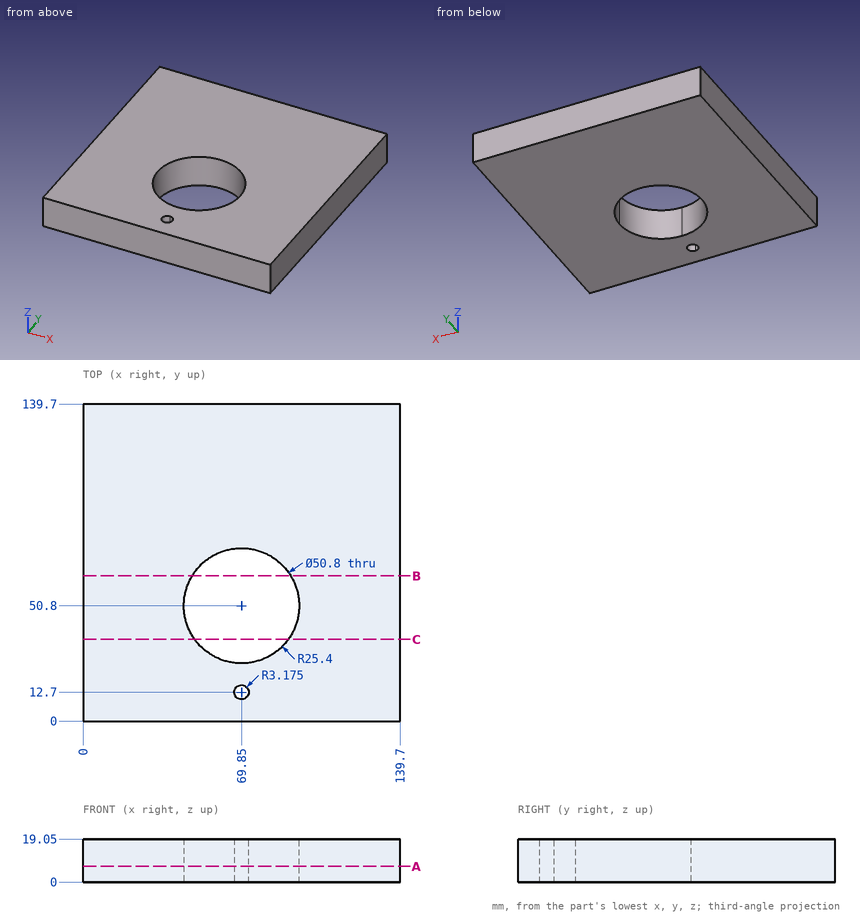
Print and shaded views of the part. All mm, measured from the part's lowest x, y and z. Round coordinates to 2 decimals unless told otherwise and drop trailing zeros. Write each loop counter-clockwise with the first axis right and the second up, starting at its lowest first coordinate (ties: lowest second). Pieces come first, ordered by that corner, then holes. Notation, with made-up numbers: M 13.5,-18.5 L 66.5,-18.5 A30 cw 66.5,18.5 Z; hole C 52.5,23.25 d3. An arc over 180 degrees is marked long. Use a Markdown table: item, result. Add a question column.
1. Drill centre lines: probe 1 along Y at (x, z) = (69.85, 13.25) (3 decimals); probe 2 along Y at (x, z) = (68, 5.5); probe 3 along X at (y, z) = (50.8, 14.5). Where is each one in solid material? Low to high.
2. Slice it at A-A on z = 7. Give the cut face in (x, y) (3 decimals).
3. Slice it at C-C on y = 36. Give the cut face in (x, z).
4. Slice it at B-B on y = 64. Give the cut face in (x, z), then the cut area to 3 significant figures.
Reply:
| question | item | result |
|---|---|---|
| 1 | probe 1 | y = 0 to 9.525, 15.875 to 25.4, 76.2 to 139.7 |
| 1 | probe 2 | y = 0 to 10.12, 15.28 to 25.47, 76.13 to 139.7 |
| 1 | probe 3 | x = 0 to 44.45, 95.25 to 139.7 |
| 2 | outline | M 0,0 L 139.7,0 L 139.7,139.7 L 0,139.7 Z; hole C 69.85,50.8 d50.8; hole C 69.85,12.7 d6.35 |
| 3 | outline | M 0,0 L 49.21,0 L 49.21,19.05 L 0,19.05 Z; M 90.49,0 L 139.7,0 L 139.7,19.05 L 90.49,19.05 Z |
| 4 | outline | M 0,0 L 48.15,0 L 48.15,19.05 L 0,19.05 Z; M 91.55,0 L 139.7,0 L 139.7,19.05 L 91.55,19.05 Z |
| 4 | area | 1,830 mm^2 |
